Source: CAD feature listing. Evaluate the final solid. Frame: model axes, mm. Face numbers are marked on the shaded views. Coordinates: 2 decimals unless noted, no trailing zeros. Write each loop counter-clockwise with the first axis right and the second up, starting at its lowest first coordinate (ties: lowest second). Pieces come first, ordered by that corner, then holes. Notation, with made-up numbers: M 63,44.5 L 110,44.5 A17 ccw 110,51.5 Z; hole C 5.25,66.25 d10. An arc over 180 degrees is marked long. Answer as CSV lines item,"result". Start each with the question number.
1. Section B-B on x = 15. Return the cut outline in (y, z), plus the area to 3 significant figures.
2. Section C-C on y = 0. Return the cut outline in (x, z).
3. Mould query, pull axis Y, two halves, no side actions, for the marked faces 1, 2, 3 and 4. Classes: pulls with the +Y half, pulls with the -Y half, needs draft (parallel to the pull), parting line crosses it, or undercut.
4. Contact query for flat-ended pins moving along their axis: pin 1 Ø3 at (x, y) = (-14.5, -1.5) entering from +Z; pin 2 Ø3 at (x, y) = (15, 0) entering from +Z. Output: stop coordinate, or through.
5. Section D-D on z = 1.5. Return the cut outline in (x, y).
6. Line query: probe 1 along X at (y, z) = (0, 2.75); probe 2 along X at (y, z) = (0, 6.85); probe 3 along Y at (x, z) = (-15, 2.8). Output: solid intervals per line, ascending. Write a range as [from, to].
7. Section A-A on z = 6.75. Return the cut outline in (x, y), plus the area to 3 significant figures.
Solid Edge part; units mm, degrees
sketch "Sketch1" plane through (0, 0, 0) normal (0, 0, 1) x (1, 0, 0)
  line L0 (-20, 6) -> (-20, -6)
  line L1 (-20, -6) -> (20, -6)
  line L2 (20, -6) -> (20, 6)
  line L3 (20, 6) -> (-20, 6)
  dimension "D1" = 20
extrude "Protrusion1" add sketch "Sketch1" along normal blind 7.7
hole "Hole_1" at (15, 0, 7.7) direction (0, 0, -1) diameter 3.6 end through all counterbore diameter 6.5 counterbore depth 4
hole "Hole1" at (-15, 0, 7.7) direction (0, 0, -1) diameter 3.6 end through all counterbore diameter 6.5 counterbore depth 4
fillet "Round_1" radius 1.5 4 edges at (20, 6, 3.85) (20, -6, 3.85) (-20, -6, 3.85) (-20, 6, 3.85)
properties material "Acrylic, high impact grade"
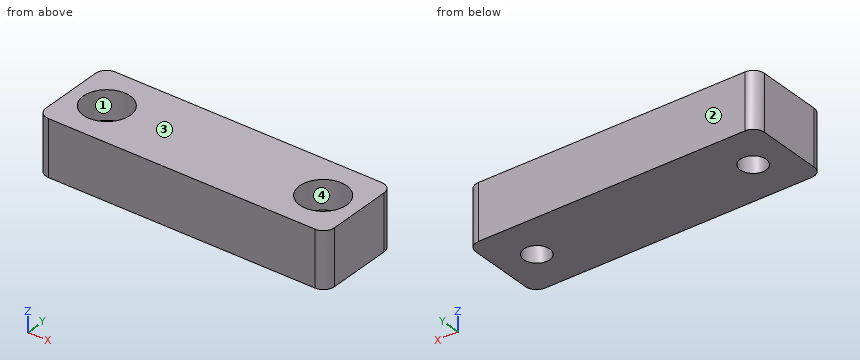
Values:
1,outline,"M -6,0 L -1.8,0 L -1.8,3.7 L -3.25,3.7 L -3.25,7.7 L -6,7.7 Z; M 1.8,0 L 6,0 L 6,7.7 L 3.25,7.7 L 3.25,3.7 L 1.8,3.7 Z"
1,area,"53.1 mm²"
2,outline,"M -20,0 L -16.8,0 L -16.8,3.7 L -18.25,3.7 L -18.25,7.7 L -20,7.7 Z; M -13.2,0 L 13.2,0 L 13.2,3.7 L 11.75,3.7 L 11.75,7.7 L -11.75,7.7 L -11.75,3.7 L -13.2,3.7 Z; M 16.8,0 L 20,0 L 20,7.7 L 18.25,7.7 L 18.25,3.7 L 16.8,3.7 Z"
3,face 1,"undercut"
3,face 2,"pulls with the +Y half"
3,face 3,"needs draft"
3,face 4,"undercut"
4,pin 1,"z = 3.7"
4,pin 2,"through"
5,outline,"M -20,-4.5 A1.5 ccw -18.5,-6 L 18.5,-6 A1.5 ccw 20,-4.5 L 20,4.5 A1.5 ccw 18.5,6 L -18.5,6 A1.5 ccw -20,4.5 Z; hole C -15,0 d3.6; hole C 15,0 d3.6"
6,probe 1,"[-20, -16.8], [-13.2, 13.2], [16.8, 20]"
6,probe 2,"[-20, -18.25], [-11.75, 11.75], [18.25, 20]"
6,probe 3,"[-6, -1.8], [1.8, 6]"
7,outline,"M -20,-4.5 A1.5 ccw -18.5,-6 L 18.5,-6 A1.5 ccw 20,-4.5 L 20,4.5 A1.5 ccw 18.5,6 L -18.5,6 A1.5 ccw -20,4.5 Z; hole C -15,0 d6.5; hole C 15,0 d6.5"
7,area,"412 mm²"
